Here's how the part is built. I have some questions about the finished solid (model axes, mm). A direction names the side the tool comes from. Round coordinates to 2 decimals unless told otherwise and drop trailing zeros. Loops run counter-clockwise (first coordinate to the right, second up) from the corner with the lowest first, then second, coordinate; pieces in that order, holes last. Notation, with made-up numbers: M 72,-21 L 88,-21 A6 ccw 88,-11 Z; hole C 81,31.25 d5. An arc over 180 degrees is marked long. Write each question's results on one line, items separated by ' | '. Start each with the question number.
```python
from build123d import *

# Parameters (mm, degrees)
SKETCH1_W                = 20
SKETCH1_H                = 25
BOSS_EXTRUDE1_DEPTH      = 20
BOSS_EXTRUDE2_DEPTH      = 20
BOSS_EXTRUDE2_DEPTH_BACK = 10
SKETCH2_R                = 10
CUT_EXTRUDE1_DEPTH       = 59.309518948
SKETCH3_W                = 10
SKETCH3_H                = 5
CUT_EXTRUDE2_DEPTH       = 54.851648071
SKETCH4_R                = 15
CUT_EXTRUDE3_DEPTH       = 10


with BuildPart() as part:
    # Sketch1 → Boss-Extrude1 (new body)
    with BuildSketch(Plane.XY):
        with Locations((10, -12.5)):
            Rectangle(SKETCH1_W, SKETCH1_H)
        with Locations((-10, -12.5)):
            Rectangle(SKETCH1_W, SKETCH1_H)
    extrude(amount=BOSS_EXTRUDE1_DEPTH)

    # Sketch1_3 → Boss-Extrude2 (add, two sides: drawn at the far end of the back side and taken through both)
    with BuildSketch(Plane.XY.offset(-BOSS_EXTRUDE2_DEPTH_BACK)):
        Polygon((20, -25), (-20, -25), (-30, -25), (-30, -40), (30, -40), (30, -25), align=None)
    extrude(amount=BOSS_EXTRUDE2_DEPTH + BOSS_EXTRUDE2_DEPTH_BACK)

    # Sketch2 → Cut-Extrude1 (cut, through all)
    with BuildSketch(Plane.XY.offset(20)):
        Circle(SKETCH2_R)
    extrude(amount=-CUT_EXTRUDE1_DEPTH, mode=Mode.SUBTRACT)

    # Sketch3 → Cut-Extrude2 (cut, through all)
    with BuildSketch(Plane(origin=(0, 0, 0), x_dir=(1, 0, 0), z_dir=(0, 1, 0))):
        with Locations((0, -17.5)):
            Rectangle(SKETCH3_W, SKETCH3_H)
    extrude(amount=-CUT_EXTRUDE2_DEPTH, mode=Mode.SUBTRACT)

    # Sketch4 → Cut-Extrude3 (cut)
    with BuildSketch(Plane.XY.offset(20)):
        Circle(SKETCH4_R)
    extrude(amount=-CUT_EXTRUDE3_DEPTH, mode=Mode.SUBTRACT)


solid = part.part
```
1. I want a section at D-D on z = 4.25. List the corners of the cut face in (x, y) for me, plus the area to 3 significant figures.
2. I want a section at B-B on x = 0. List the corners of the cut face in (y, z) for me.
3. I want a section at A-A on z = 18. List the corners of the cut face in (x, y) for me.
4. I need wall thicknesses on line 1 along Y through (x, z) = (24, 2.25); line 2 along X through (y, z) = (-4.5, 9.25); line 3 along X through (y, z) = (-22, 9.75). Which ranges of each line are inside material? Lowest first, please.
5. For pin 1 (4 mm diameter, centred on y = -23.5, z = 16.5, fed in from +X); pin 2 (2 mm diameter, centred on y = -22, z = 1, fed in from +X); pin 3 (12.5 mm diameter, centred on x = -2, y = -12, fed in from -Z); pin 4 (12 mm diameter, centred on y = -15, z = 15.5, fed in from -X), each with a flat end and sliding along its axis, tell me the tip position at first contact or that it passes through.
6. If we mould it in two halves opening along X, with no side actions, what happens to faces 6 (the face through (0, -15, 14)), 7 (the face through (-16, 0, 8)), 8 (the face through (-20, -13, 10))? For each: released by +X, released by -X, zero draft, split by the parting line, or undercut.
7. Which directions (+Z, -Z, +X, -X, +Y, -Y) give clear straight access to the entire face, cutting with the end or side of a thin tool? Please do faces 1 (the face through (0, -11, 10)), 2 (the face through (-5, -27, 18)), 3 (the face through (-30, -32, 5)), 4 (the face through (20, -13, 10)), 5 (the face through (0, -15, 0)).
8. I want a section at C-C on y = -26.5. List the corners of the cut face in (x, z) for me.
Outcome:
1) outline: M -30,-40 L 30,-40 L 30,-25 L 20,-25 L 20,0 L 10,0 A10 cw -10,0 L -20,0 L -20,-25 L -30,-25 Z | area: 1,740 mm2
2) outline: M -40,-10 L -25,-10 L -25,0 L -10,0 L -10,10 L -15,10 L -15,15 L -40,15 Z
3) outline: M -30,-40 L -5,-40 L -5,-14.14 A15 cw -15,0 L -20,0 L -20,-25 L -30,-25 Z; M 5,-40 L 30,-40 L 30,-25 L 20,-25 L 20,0 L 15,0 A15 cw 5,-14.14 Z
4) line 1: -40 to -25 | line 2: -20 to -8.93, 8.93 to 20 | line 3: -20 to 20
5) pin 1: x = 30 | pin 2: x = 20 | pin 3: z = 0 | pin 4: x = -20
6) face 6: undercut | face 7: zero draft | face 8: released by -X
7) face 1: +Z, +Y | face 2: +Z, +Y, -Y | face 3: +Z, -Z, -X, +Y, -Y | face 4: +Z, -Z, +X, +Y | face 5: -Z, +X, -X, +Y
8) outline: M -30,-10 L 30,-10 L 30,20 L 5,20 L 5,15 L -5,15 L -5,20 L -30,20 Z
